Read the model definition and answer for the solid it produces. Units are mm, in the model's axes. Give positions to 0.01 mm unless a question says otherwise; leave off trailing zeros. Loops run counter-clockwise (first coordinate to the right, second up) from the corner with the lowest first, then second, coordinate; pieces in that order, holes last. Notation, with made-up numbers: (-29, 36) - (-22, 36) arc R25 ccw to (-22, 52) - close; hole circle Ø4 at (38, -27). An arc over 180 degrees is marked (long way). Write item = value, one per line. Start each with the question number.
from build123d import *

# Parameters (mm, degrees)
SKETCH1_W           = 32
SKETCH1_H           = 32
SKETCH1_R           = 1.04775
BOSS_EXTRUDE1_DEPTH = 1.6002
BOSS_EXTRUDE2_DEPTH = 5.1308
FILLET1_R           = 2.1
FILLET2_R           = 1.905
SKETCH3_R           = 7.5946
BOSS_EXTRUDE3_DEPTH = 16.129


# Read off the part's stored shape, not the designer's step: Extrude-Thin2
with BuildPart() as part:
    # Sketch1 → Boss-Extrude1 (new body)
    with BuildSketch(Plane(origin=(0, 0, 0), x_dir=(1, 0, 0), z_dir=(0, 1, 0))):
        Rectangle(SKETCH1_W, SKETCH1_H)
        with Locations(Location((13.7500106, 13.7500106, 0), (0, 0, 270))):
            Circle(SKETCH1_R, mode=Mode.SUBTRACT)
        with Locations(Location((-13.7500106, 13.7500106, 0), (0, 0, 270))):
            Circle(SKETCH1_R, mode=Mode.SUBTRACT)
        with Locations(Location((-13.75, -13.7500106, 0), (0, 0, 270))):
            Circle(SKETCH1_R, mode=Mode.SUBTRACT)
        with Locations(Location((13.7500106, -13.7500106, 0), (0, 0, 270))):
            Circle(SKETCH1_R, mode=Mode.SUBTRACT)
    extrude(amount=BOSS_EXTRUDE1_DEPTH)

    # Sketch2 → Boss-Extrude2 (add)
    with BuildSketch(Plane(origin=(0, 1.6002, 0), x_dir=(1, 0, 0), z_dir=(0, 1, 0))):
        Polygon((-10.033, 9.525), (10.033, 9.525), (10.033, 2.2733), (13.2334, 2.2733), (13.2334, -2.2733), (10.033, -2.2733), (10.033, -9.525), (-10.033, -9.525), (-10.033, -2.2733), (-13.2334, -2.2733), (-13.2334, 2.2733), (-10.033, 2.2733), align=None)
    extrude(amount=BOSS_EXTRUDE2_DEPTH)

    # Fillet1
    fillet1_edges = [part.edges().sort_by_distance(p)[0] for p in [
        (-16, 0.8001, -16),
        (16, 0.8001, -16),
        (16, 0.8001, 16),
        (-16, 0.8001, 16),
    ]]
    fillet(fillet1_edges, radius=FILLET1_R)

    # Fillet2
    fillet2_edges = [part.edges().sort_by_distance(p)[0] for p in [
        (-10.033, 4.1656, -9.525),
        (-13.2334, 4.1656, -2.2733),
        (-13.2334, 4.1656, 2.2733),
        (-10.033, 4.1656, 9.525),
        (10.033, 4.1656, 9.525),
        (13.2334, 4.1656, 2.2733),
        (13.2334, 4.1656, -2.2733),
        (10.033, 4.1656, -9.525),
    ]]
    fillet(fillet2_edges, radius=FILLET2_R)

    # Sketch3 → Boss-Extrude3 (add)
    with BuildSketch(Plane(origin=(0, 6.731, 0), x_dir=(1, 0, 0), z_dir=(0, 1, 0))):
        with Locations(Location((0, 0, 0), (0, 0, 90))):
            Circle(SKETCH3_R)
    extrude(amount=BOSS_EXTRUDE3_DEPTH)

    # Extrude-Thin2 outline → Extrude-Thin2 (revolve)
    with BuildSketch(Plane.XY):
        Polygon((0, 175.26), (0, 24.764601785), (3.048, 22.86), (3.175, 22.86), (4.3815, 23.613904873), (5.588, 22.86), (5.715, 22.86), (249.605982226, 175.26), align=None)
    revolve(axis=Axis((0, 0, 0), (0, 1, 0)))


solid = part.part
1. Given P1, Ø4, axis at y = 5, z = -4.5, coming from the -X side; P2, Ø0.6, axis at y = 4.5, z = 0, coming from the -X side; P3, Ø0.6, axis at x = -11, y = 4.5, coming from the -Z side, each flat-ended and moving along its own axis, determine where each tip first touches the part or whether it passes through.
2. A cutting plane is placed at B-B on y = 157. Give the vertices of the cut face in (x, z).
3. For a pull along Y with two mould halves and no side action, classify faces 1 (the flat face through (0, 0, 0)), 2 (the flat face through (-3, 175.26, -3)), 3 (the flat face through (4, 22.86, 0)) as released by +Y, released by -Y, zero draft, split by the parting line, or undercut.
4. A cutting plane is placed at A-A on y = 113.5. Give the vertices of the cut face in (x, z).
5. Consider line 1 along Y through (x, z) = (-31, 183); line 2 along Y through (x, z) = (-228, -36); line 3 along X through (y, z) = (71.5, 46). Determine where each line is inside the solid, lowest interval first. Write a range as [from, to].
Reply:
q1.P1 = -10.03
q1.P2 = -13.23
q1.P3 = -2.27
q2.outline = circle Ø440.77 at (0, 0)
q3.face_1 = released by -Y
q3.face_2 = released by +Y
q3.face_3 = undercut
q4.outline = circle Ø301.54 at (0, 0)
q5.line_1 = [135.27, 175.26]
q5.line_2 = [163.52, 175.26]
q5.line_3 = [-69.75, 69.75]
